```python
from build123d import *

# Parameters (mm, degrees)
SKETCH1_W           = 20.63
SKETCH1_H           = 43.7
BOSS_EXTRUDE1_DEPTH = 1.5
SKETCH2_R           = 1.5
CUT_EXTRUDE1_DEPTH  = 1.5
BOSS_EXTRUDE2_DEPTH = 1.9
SKETCH4_R           = 4
BOSS_EXTRUDE3_DEPTH = 10.04
SKETCH5_W           = 12.12
SKETCH5_H           = 12.12
BOSS_EXTRUDE4_DEPTH = 7.9


with BuildPart() as part:
    # Sketch1 → Boss-Extrude1 (new body)
    with BuildSketch(Plane(origin=(0, 0, 0), x_dir=(1, 0, 0), z_dir=(0, 1, 0))):
        Rectangle(SKETCH1_W, SKETCH1_H)
    extrude(amount=BOSS_EXTRUDE1_DEPTH)

    # Sketch2 → Cut-Extrude1 (cut)
    with BuildSketch(Plane(origin=(0, 1.5, 0), x_dir=(1, 0, 0), z_dir=(0, 1, 0))):
        with Locations((7.605, 14.68)):
            Circle(SKETCH2_R)
        with Locations((-7.315, -15.31)):
            Circle(SKETCH2_R)
    extrude(amount=-CUT_EXTRUDE1_DEPTH, mode=Mode.SUBTRACT)

    # Sketch3 → Boss-Extrude2 (add)
    with BuildSketch(Plane(origin=(0, 1.5, 0), x_dir=(1, 0, 0), z_dir=(0, 1, 0))):
        Polygon((0, -21.66), (-4.15, -21.66), (-4.15, -13.36), (4.15, -13.36), (4.15, -21.66), align=None)
    boss_extrude2 = extrude(amount=BOSS_EXTRUDE2_DEPTH)

    # Sketch4 → Boss-Extrude3 (add)
    with BuildSketch(Plane(origin=(0, 3.4, 0), x_dir=(1, 0, 0), z_dir=(0, 1, 0))):
        with Locations((0, -17.51)):
            Circle(SKETCH4_R)
    boss_extrude3 = extrude(amount=BOSS_EXTRUDE3_DEPTH)

    # Mirror1: Boss-Extrude2, Boss-Extrude3 across plane
    add(boss_extrude2.mirror(Plane.XY))
    add(boss_extrude3.mirror(Plane.XY))

    # Sketch5 → Boss-Extrude4 (add)
    with BuildSketch(Plane(origin=(0, 1.5, 0), x_dir=(1, 0, 0), z_dir=(0, 1, 0))):
        with Locations((2.425, 6.75)):
            Rectangle(SKETCH5_W, SKETCH5_H)
    extrude(amount=BOSS_EXTRUDE4_DEPTH)


solid = part.part
```
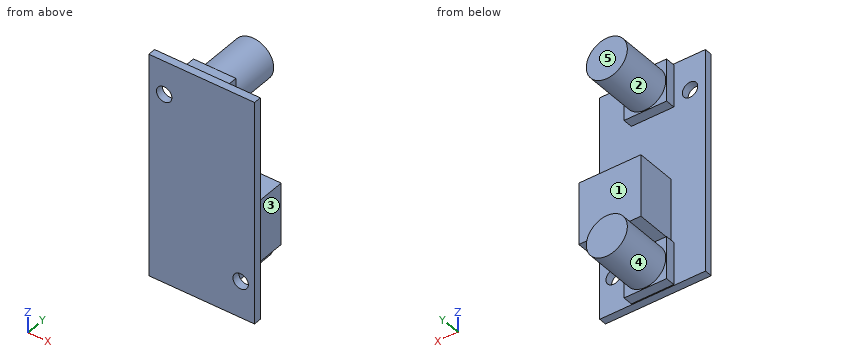
CAD build for the part. Positions are in the model's coordinates, mm. Face numbers are marked on the shaded views. A direction names the side the tool comes from. Coordinates: 2 decimals unless noted, no trailing zeros. Write each loop counter-clockwise with the first axis right and the second up, starting at its lowest first coordinate (ties: lowest second). Pieces come first, ordered by that corner, then holes. Notation, with made-up numbers: (-14, -30.75) -> (22, -30.75) arc R24 ccw to (22, -9.75) -> close; hole circle Ø6 at (31, 4.25). An arc over 180 degrees is marked (long way). Use CSV: the item, a comma, the result in double quotes. Start each with the question number.
Item 1: Wall check: probe 1 along X at (y, z) = (0.65, 15.31) (3 decimals); probe 2 along Z at (x, y) = (-0.5, 5.5); probe 3 along Z at (x, y) = (1.25, 2). Give the ranges that are in metal, low to high.
Item 2: Band-saw the part on A-A, the plane y = 2. Write the cut outline in (x, z) (3 decimals), plus the area to 3 significant figures.
Item 3: Band-saw the part on C-C, the plane z = 16. Write the cut outline in (x, y) (3 decimals).
Item 4: Drop flat-ended pins along their axis: P1, Ø6.5, axis at y = 4.5, z = -7, coming from the +X side (3 decimals); P2, Ø1, axis at x = -4, y = 2.5, coming from the -Z side; P3, Ø4, axis at y = 5.5, z = -9, coming from the -X side (3 decimals); P4, Ø2, axis at x = -2, z = -7.5, coming from the +Y side. Give the stop position or say it passes through.
Item 5: Band-saw the part on D-D, the plane x = 0. Write the cut outline in (y, z).
Item 6: Two-plate mould, pull along Z, no slides. Class the marked faces 4 and 5: +Z half, -Z half, draft (parallel to the pull), parting line (faces both ways), or undercut.
Item 7: Band-saw the part on B-B, the plane x = -7.75. Write the cut outline in (y, z), plus the area to 3 significant figures.
Item 8: Tool access for the marked faces 1, 2 and 3: list every direction of +Z, -Z, +X, -X, +Y, -Y with a clear straight run to the whole face (end or side of a thin tool).
Response values:
1,probe 1,"x = -10.315 to -8.815, -5.815 to 10.315"
1,probe 2,"z = -21.48 to -13.54, -12.81 to -0.69, 13.54 to 21.48"
1,probe 3,"z = -21.66 to -13.36, -12.81 to -0.69, 13.36 to 21.66"
2,outline,"(-4.15, -21.66) -> (4.15, -21.66) -> (4.15, -13.36) -> (-4.15, -13.36) -> close; (-4.15, 13.36) -> (4.15, 13.36) -> (4.15, 21.66) -> (-4.15, 21.66) -> close; (-3.635, -12.81) -> (8.485, -12.81) -> (8.485, -0.69) -> (-3.635, -0.69) -> close"
2,area,"285 mm2"
3,outline,"(-10.315, 0) -> (-8.647, 0) -> (-8.647, 1.5) -> (-10.315, 1.5) -> close; (-5.983, 0) -> (10.315, 0) -> (10.315, 1.5) -> (4.15, 1.5) -> (4.15, 3.4) -> (3.704, 3.4) -> (3.704, 13.44) -> (-3.704, 13.44) -> (-3.704, 3.4) -> (-4.15, 3.4) -> (-4.15, 1.5) -> (-5.983, 1.5) -> close"
4,P1,"stops at x = 10.315"
4,P2,"stops at z = -21.66"
4,P3,"stops at x = -3.635"
4,P4,"stops at y = 9.4"
5,outline,"(0, -21.85) -> (1.5, -21.85) -> (1.5, -21.66) -> (3.4, -21.66) -> (3.4, -21.51) -> (13.44, -21.51) -> (13.44, -13.51) -> (3.4, -13.51) -> (3.4, -13.36) -> (1.5, -13.36) -> (1.5, -12.81) -> (9.4, -12.81) -> (9.4, -0.69) -> (1.5, -0.69) -> (1.5, 13.36) -> (3.4, 13.36) -> (3.4, 13.51) -> (13.44, 13.51) -> (13.44, 21.51) -> (3.4, 21.51) -> (3.4, 21.66) -> (1.5, 21.66) -> (1.5, 21.85) -> (0, 21.85) -> close"
6,face 4,"undercut"
6,face 5,"draft"
7,outline,"(0, -21.85) -> (1.5, -21.85) -> (1.5, 13.87) -> (0, 13.87) -> close; (0, 16.75) -> (1.5, 16.75) -> (1.5, 21.85) -> (0, 21.85) -> close"
7,area,"61.2 mm2"
8,face 1,"+X, -X, +Y"
8,face 2,"+Y"
8,face 3,"+Z, -Z, +X, +Y"
